Could you check a few things on this model? Use its own coordinates, in mm. Face numbers are marked on the shaded views. Round coordinates to 2 decimals unless told otherwise and drop trailing zeros. Order: outer loops, then holes, each group sorted by start corner. A loop starts at its lowest first (then second) coordinate and runs counter-clockwise, first axis right, second up. Notation, with made-up numbers: (21.25, -28) - (34.25, -28) arc R20 ccw to (34.25, -5) - close; hole circle Ø7 at (23.25, 3.25). An arc over 180 degrees is marked (long way). Use one line per item in the form item = value.
from build123d import *

# Parameters (mm, degrees)
M6_TAPPED_HOLE1_D     = 5
M6_TAPPED_HOLE1_DEPTH = 20
M6_TAPPED_HOLE1_TIP   = 1.502151548
CHAMFER1_SIZE         = 1.25095704
SKETCH8_R             = 10.8
SKETCH8_R_2           = 6
CUT_EXTRUDE2_DEPTH    = 0.5
CHAMFER2_SIZE         = 0.5
CUT_EXTRUDE3_START    = -2
CUT_EXTRUDE3_DEPTH    = 46.048166808


# Some blends are built 0.0001 mm under size
with BuildPart() as part:
    # Sketch1 → Revolve1 (revolve)
    with BuildSketch(Plane.XY, mode=Mode.PRIVATE) as revolve1_sk:
        with BuildLine():
            Line((0, 0), (48, 0))
            ThreePointArc((48, 0), (47.749466448, 5.423098745), (47, 10.8))
            Line((47, 10.8), (44, 10.8))
            Line((44, 10.8), (44, 4))
            Line((44, 4), (0, 4))
            Line((0, 4), (0, 0))
        make_face()
    revolve(revolve1_sk.sketch.rotate(Axis((0, 0, 0), (1, 0, 0)), 90), axis=Axis((0, 0, 0), (1, 0, 0)))

    # M6 Tapped Hole1
    with Locations(Plane.ZY):
        with Locations((0, 0)):
            Hole(M6_TAPPED_HOLE1_D / 2, depth=M6_TAPPED_HOLE1_DEPTH)
            with Locations((0, 0, -(M6_TAPPED_HOLE1_DEPTH + M6_TAPPED_HOLE1_TIP / 2))):  # 118° drill point
                Cone(0, M6_TAPPED_HOLE1_D / 2, M6_TAPPED_HOLE1_TIP, mode=Mode.SUBTRACT)

    # Chamfer1
    # the kernel refuses this chamfer: 1.25095704, 1 mm, written as the material it takes off along each edge
    with BuildSketch(Plane(origin=(47, 0, 0), x_dir=(0, 0, 1), z_dir=(0, 1, 0))) as chamfer1_piece_1:
        with BuildLine():
            Line((9.823683565, 0.173858651), (10.8, -CHAMFER1_SIZE))
            Line((10.8, -CHAMFER1_SIZE), (10.8, 0))
            ThreePointArc((10.8, 0), (10.294942592, 0.092058822), (9.823683565, 0.173858651))
        make_face()
    revolve(axis=Axis((47, 0, 0), (1, 0, 0)), mode=Mode.SUBTRACT)

    # Sketch8 → Cut-Extrude2 (cut)
    with BuildSketch(Plane.ZY.offset(-44)):
        Circle(SKETCH8_R)
        Circle(SKETCH8_R_2, mode=Mode.SUBTRACT)
    extrude(amount=-CUT_EXTRUDE2_DEPTH, mode=Mode.SUBTRACT)

    # Chamfer2
    chamfer2_edges = [part.edges().sort_by_distance(p)[0] for p in [
        (44, 0, -6),
    ]]
    chamfer(chamfer2_edges, length=CHAMFER2_SIZE - 0.0001)  # a hair under: the kernel refuses the full size

    # Sketch9 → Cut-Extrude3 (cut, through all)
    with BuildSketch(Plane.ZY.offset(-44.5).offset(CUT_EXTRUDE3_START)):
        Polygon((1.154700538, -2), (2.309401077, 0), (1.154700538, 2), (-1.154700538, 2), (-2.309401077, 0), (-1.154700538, -2), align=None)
    extrude(amount=-CUT_EXTRUDE3_DEPTH, mode=Mode.SUBTRACT)


solid = part.part
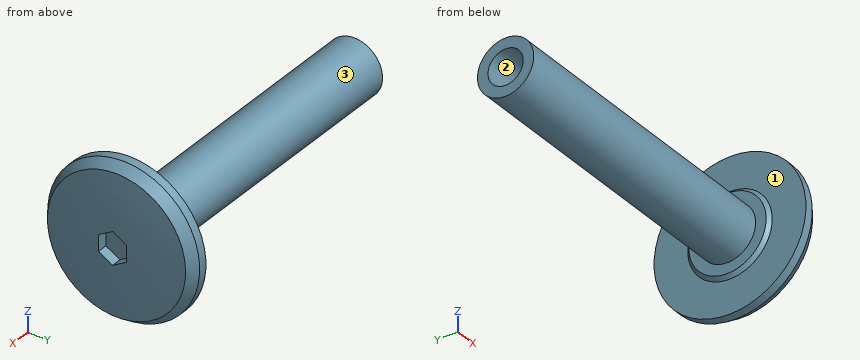
Item 1: If we mould it in two halves opening along Z, with no side actions, what happens to the marked faces 1, 2 and 3? For each: released by +Z, released by -Z, zero draft, split by the parting line, or undercut.
Found:
face_1 = zero draft
face_2 = undercut
face_3 = split by the parting line
Item 2: Imagine slicing it at B-B on x = 13.5. Please give me the cut outline in (y, z), plus the area to 3 significant figures.
Found:
outline = circle Ø8 at (0, 0); hole circle Ø5 at (0, 0)
area = 30.6 mm2
Item 3: Will these pins go through, and if not, where does the flat tip stop? P1, Ø5, axis at x = 5.5, z = -1.5, coming from the -Y side; P2, Ø3, axis at y = 0, z = 0, coming from the +X side; P3, Ø1.2, axis at x = 47, z = 0, coming from the -Y side; P4, Ø12, axis at y = -4.5, z = -6.5, coming from the -X side.
Found:
P1 = -4
P2 = 46.5
P3 = -10.35
P4 = 0
Item 4: I need wall thicknesses on L1, parallel to Y at x = 14.5, z = 0; L2, parallel to Z at x = 24, y = 0.25; L3, parallel to X at y = 7, z = 7.5. Which ranges of each line are inside material? Lowest first, please.
Found:
L1 = -4 to -2.5, 2.5 to 4
L2 = -3.99 to 3.99
L3 = 44.5 to 46.54
Item 5: Imagine slicing it at A-A on x = 38.5. Please give me the cut outline in (y, z).
Found:
outline = circle Ø8 at (0, 0)
